from build123d import *

# Parameters (mm, degrees)
SKETCH1_W           = 167.64
SKETCH1_H           = 167.64
BOSS_EXTRUDE1_DEPTH = 6.35
SKETCH2_R           = 19.725818268
BOSS_EXTRUDE2_DEPTH = 6.35
SKETCH3_R           = 1.6
CUT_EXTRUDE1_DEPTH  = 10
SKETCH5_R           = 1.6
CUT_EXTRUDE3_DEPTH  = 119.709339565
CIRPATTERN2_COUNT   = 4
SKETCH6_R           = 1.6
CUT_EXTRUDE4_DEPTH  = 119.709339565
CIRPATTERN3_COUNT   = 4
SKETCH7_R           = 5
CUT_EXTRUDE5_DEPTH  = 119.709339565
CIRPATTERN4_COUNT   = 4
FILLET1_R           = 10


with BuildPart() as part:
    # Sketch1 → Boss-Extrude1 (new body)
    with BuildSketch(Plane(origin=(0, 0, 0), x_dir=(1, 0, 0), z_dir=(0, 1, 0))):
        Rectangle(SKETCH1_W, SKETCH1_H)
    extrude(amount=BOSS_EXTRUDE1_DEPTH)

    # Sketch2 → Boss-Extrude2 (add)
    with BuildSketch(Plane(origin=(0, 6.35, 0), x_dir=(1, 0, 0), z_dir=(0, 1, 0))):
        with Locations(Location((0, 0, 0), (0, 0, 270))):
            Circle(SKETCH2_R)
    extrude(amount=BOSS_EXTRUDE2_DEPTH)

    # Sketch3 → Cut-Extrude1 (cut)
    with BuildSketch(Plane(origin=(0, 6.35, 0), x_dir=(1, 0, 0), z_dir=(0, 1, 0))):
        with Locations(Location((5.59999998, 75.42, 0), (0, 0, 270))):
            Circle(SKETCH3_R)
        with Locations(Location((-25.60000002, 75.42, 0), (0, 0, 270))):
            Circle(SKETCH3_R)
        with Locations(Location((5.59999998, 69.02, 0), (0, 0, 270))):
            Circle(SKETCH3_R)
        with Locations(Location((-25.60000002, 69.02, 0), (0, 0, 270))):
            Circle(SKETCH3_R)
        with Locations(Location((5.59999998, 62.62, 0), (0, 0, 270))):
            Circle(SKETCH3_R)
        with Locations(Location((-25.60000002, 62.62, 0), (0, 0, 270))):
            Circle(SKETCH3_R)
        with Locations(Location((5.59999998, 56.22, 0), (0, 0, 270))):
            Circle(SKETCH3_R)
        with Locations(Location((-25.60000002, 56.22, 0), (0, 0, 270))):
            Circle(SKETCH3_R)
        with Locations(Location((5.59999998, 49.82, 0), (0, 0, 270))):
            Circle(SKETCH3_R)
        with Locations(Location((-25.60000002, 49.82, 0), (0, 0, 270))):
            Circle(SKETCH3_R)
        with Locations(Location((5.59999998, 43.42, 0), (0, 0, 270))):
            Circle(SKETCH3_R)
        with Locations(Location((-25.60000002, 43.42, 0), (0, 0, 270))):
            Circle(SKETCH3_R)
        with Locations(Location((5.59999998, 37.02, 0), (0, 0, 270))):
            Circle(SKETCH3_R)
        with Locations(Location((-25.60000002, 37.02, 0), (0, 0, 270))):
            Circle(SKETCH3_R)
        with Locations(Location((75.42, -5.59999998, 0), (0, 0, 270))):
            Circle(SKETCH3_R)
        with Locations(Location((75.42, 25.60000002, 0), (0, 0, 270))):
            Circle(SKETCH3_R)
        with Locations(Location((69.02, -5.59999998, 0), (0, 0, 270))):
            Circle(SKETCH3_R)
        with Locations(Location((62.62, -5.59999998, 0), (0, 0, 270))):
            Circle(SKETCH3_R)
        with Locations(Location((56.22, -5.59999998, 0), (0, 0, 270))):
            Circle(SKETCH3_R)
        with Locations(Location((49.82, -5.59999998, 0), (0, 0, 270))):
            Circle(SKETCH3_R)
        with Locations(Location((43.42, -5.59999998, 0), (0, 0, 270))):
            Circle(SKETCH3_R)
        with Locations(Location((37.02, -5.59999998, 0), (0, 0, 270))):
            Circle(SKETCH3_R)
        with Locations(Location((69.02, 25.60000002, 0), (0, 0, 270))):
            Circle(SKETCH3_R)
        with Locations(Location((62.62, 25.60000002, 0), (0, 0, 270))):
            Circle(SKETCH3_R)
        with Locations(Location((56.22, 25.60000002, 0), (0, 0, 270))):
            Circle(SKETCH3_R)
        with Locations(Location((49.82, 25.60000002, 0), (0, 0, 270))):
            Circle(SKETCH3_R)
        with Locations(Location((43.42, 25.60000002, 0), (0, 0, 270))):
            Circle(SKETCH3_R)
        with Locations(Location((37.02, 25.60000002, 0), (0, 0, 270))):
            Circle(SKETCH3_R)
        with Locations(Location((-5.59999998, -75.42, 0), (0, 0, 270))):
            Circle(SKETCH3_R)
        with Locations(Location((25.60000002, -75.42, 0), (0, 0, 270))):
            Circle(SKETCH3_R)
        with Locations(Location((-5.59999998, -69.02, 0), (0, 0, 270))):
            Circle(SKETCH3_R)
        with Locations(Location((-5.59999998, -62.62, 0), (0, 0, 270))):
            Circle(SKETCH3_R)
        with Locations(Location((-5.59999998, -56.22, 0), (0, 0, 270))):
            Circle(SKETCH3_R)
        with Locations(Location((-5.59999998, -49.82, 0), (0, 0, 270))):
            Circle(SKETCH3_R)
        with Locations(Location((-5.59999998, -43.42, 0), (0, 0, 270))):
            Circle(SKETCH3_R)
        with Locations(Location((-5.59999998, -37.02, 0), (0, 0, 270))):
            Circle(SKETCH3_R)
        with Locations(Location((25.60000002, -69.02, 0), (0, 0, 270))):
            Circle(SKETCH3_R)
        with Locations(Location((25.60000002, -62.62, 0), (0, 0, 270))):
            Circle(SKETCH3_R)
        with Locations(Location((25.60000002, -56.22, 0), (0, 0, 270))):
            Circle(SKETCH3_R)
        with Locations(Location((25.60000002, -49.82, 0), (0, 0, 270))):
            Circle(SKETCH3_R)
        with Locations(Location((25.60000002, -43.42, 0), (0, 0, 270))):
            Circle(SKETCH3_R)
        with Locations(Location((25.60000002, -37.02, 0), (0, 0, 270))):
            Circle(SKETCH3_R)
        with Locations(Location((-75.42, 5.59999998, 0), (0, 0, 270))):
            Circle(SKETCH3_R)
        with Locations(Location((-75.42, -25.60000002, 0), (0, 0, 270))):
            Circle(SKETCH3_R)
        with Locations(Location((-69.02, 5.59999998, 0), (0, 0, 270))):
            Circle(SKETCH3_R)
        with Locations(Location((-62.62, 5.59999998, 0), (0, 0, 270))):
            Circle(SKETCH3_R)
        with Locations(Location((-56.22, 5.59999998, 0), (0, 0, 270))):
            Circle(SKETCH3_R)
        with Locations(Location((-49.82, 5.59999998, 0), (0, 0, 270))):
            Circle(SKETCH3_R)
        with Locations(Location((-43.42, 5.59999998, 0), (0, 0, 270))):
            Circle(SKETCH3_R)
        with Locations(Location((-37.02, 5.59999998, 0), (0, 0, 270))):
            Circle(SKETCH3_R)
        with Locations(Location((-69.02, -25.60000002, 0), (0, 0, 270))):
            Circle(SKETCH3_R)
        with Locations(Location((-62.62, -25.60000002, 0), (0, 0, 270))):
            Circle(SKETCH3_R)
        with Locations(Location((-56.22, -25.60000002, 0), (0, 0, 270))):
            Circle(SKETCH3_R)
        with Locations(Location((-49.82, -25.60000002, 0), (0, 0, 270))):
            Circle(SKETCH3_R)
        with Locations(Location((-43.42, -25.60000002, 0), (0, 0, 270))):
            Circle(SKETCH3_R)
        with Locations(Location((-37.02, -25.60000002, 0), (0, 0, 270))):
            Circle(SKETCH3_R)
    extrude(amount=-CUT_EXTRUDE1_DEPTH, mode=Mode.SUBTRACT)

    # Sketch5 → Cut-Extrude3 (cut, through all)
    with BuildSketch(Plane(origin=(0, 6.35, 0), x_dir=(1, 0, 0), z_dir=(0, 1, 0))):
        with Locations(Location((-69.75, 58.89, 0), (0, 0, 270))):
            Circle(SKETCH5_R)
        with Locations(Location((-58.89, 69.75, 0), (0, 0, 270))):
            Circle(SKETCH5_R)
    cut_extrude3 = extrude(amount=-CUT_EXTRUDE3_DEPTH, mode=Mode.SUBTRACT)

    # CirPattern2: Cut-Extrude3 ×4 about axis
    cirpattern2_axis = Axis((0, 0, 0), (0, 1, 0))
    for i in range(1, CIRPATTERN2_COUNT):
        add(cut_extrude3.rotate(cirpattern2_axis, i * 360 / CIRPATTERN2_COUNT), mode=Mode.SUBTRACT)

    # Sketch6 → Cut-Extrude4 (cut, through all)
    with BuildSketch(Plane(origin=(0, 6.35, 0), x_dir=(1, 0, 0), z_dir=(0, 1, 0))):
        with Locations(Location((-44.426601718, 73.213398282, 0), (0, 0, 270))):
            Circle(SKETCH6_R)
        with Locations(Location((-73.213398282, 44.426601718, 0), (0, 0, 270))):
            Circle(SKETCH6_R)
    cut_extrude4 = extrude(amount=-CUT_EXTRUDE4_DEPTH, mode=Mode.SUBTRACT)

    # CirPattern3: Cut-Extrude4 ×4 about axis
    cirpattern3_axis = Axis((0, 0, 0), (0, 1, 0))
    for i in range(1, CIRPATTERN3_COUNT):
        add(cut_extrude4.rotate(cirpattern3_axis, i * 360 / CIRPATTERN3_COUNT), mode=Mode.SUBTRACT)

    # Sketch7 → Cut-Extrude5 (cut, through all)
    with BuildSketch(Plane(origin=(0, 6.35, 0), x_dir=(1, 0, 0), z_dir=(0, 1, 0))):
        with Locations(Location((48.82, 48.82, 0), (0, 0, 270))):
            Circle(SKETCH7_R)
    cut_extrude5 = extrude(amount=-CUT_EXTRUDE5_DEPTH, mode=Mode.SUBTRACT)

    # CirPattern4: Cut-Extrude5 ×4 about axis
    cirpattern4_axis = Axis((0, 0, 0), (0, 1, 0))
    for i in range(1, CIRPATTERN4_COUNT):
        add(cut_extrude5.rotate(cirpattern4_axis, i * 360 / CIRPATTERN4_COUNT), mode=Mode.SUBTRACT)

    # Fillet1
    fillet1_edges = [part.edges().sort_by_distance(p)[0] for p in [
        (83.82, 3.175, 83.82),
        (-83.82, 3.175, 83.82),
        (-83.82, 3.175, -83.82),
        (83.82, 3.175, -83.82),
    ]]
    fillet(fillet1_edges, radius=FILLET1_R)


solid = part.part
Model file for the job. Use its own axes, mm. A direction names the side the tool comes from. Give positions to 0.01 mm unless a question says otherwise; leave off trailing zeros. Loops run counter-clockwise (first coordinate to the right, second up) from the corner with the lowest first, then second, coordinate; pieces in that order, holes last.
1) Pull direction Z, two halves, no side cores. Call faces 1 (the cylindrical face through (46.132, 3.219, 53.036)), 2 (the flat face through (83.82, 3, 1)), 3 (the flat face through (-1, 3, -83.82)): +Z half, -Z half, draft (parallel to the pull), parting line (faces both ways), or undercut.
2) Flat gauge pins, fed straight in: pin 1 Ø1.9 at (x, z) = (-56.22, -5.6) entering from +Y; pin 2 Ø6 at (y, z) = (9, 23.5) entering from -X; pin 3 Ø5 at (x, z) = (25.6, 62.62) entering from +Y. Where does each tip first touch, or does it go through?
3) Saw through at C-C (z = -33). Write the cut outline in (x, y), plus the area to 3 significant figures.
4) Wall check: line 1 (X direction, y = 3.25, z = 75.42); line 2 (Z direction, x = 53, y = 3); line 3 (X direction, y = 10.25, z = 0.5). Give the ranges that are in metal, low to high.
5) Tool access for faces 4 (the cylindrical face through (5.925, 9.481, 18.815)), 5 (the cylindrical face through (-46.132, 3.219, -53.036)): list every direction of +Z, -Z, +X, -X, +Y, -Y with a clear straight run to the whole face (end or side of a thin tool).
6) Saw through at B-B (y = 8.75). Write the cut outline in (x, z).
7) Saw through at A-A (z = -11.5). Write the cut outline in (x, y).
Answer block:
1. face 1: undercut
1. face 2: draft
1. face 3: -Z half
2. pin 1: passes through
2. pin 2: stops at x = -83.82
2. pin 3: stops at y = 6.35
3. outline: (-83.82, 0) - (83.82, 0) - (83.82, 6.35) - (-83.82, 6.35) - close
3. area: 1,060 mm2
4. line 1: x = -83.69 to -7.2, -4 to 24, 27.2 to 83.69
4. line 2: z = -83.82 to -51.56, -46.08 to 46.08, 51.56 to 83.82
4. line 3: x = -19.72 to 19.72
5. face 4: +Y
5. face 5: +Y, -Y
6. outline: circle Ø39.45 at (0, 0)
7. outline: (-83.82, 0) - (83.82, 0) - (83.82, 6.35) - (16.03, 6.35) - (16.03, 12.7) - (-16.03, 12.7) - (-16.03, 6.35) - (-83.82, 6.35) - close
